The model under review builds one solid part; all positions refer to its coordinate system, in mm. Face numbers are marked on the shaded views. A direction names the side the tool comes from. Round coordinates to 2 decimals unless told otherwise and drop trailing zeros. Loops run counter-clockwise (first coordinate to the right, second up) from the corner with the lowest first, then second, coordinate; pieces in that order, holes last. Notation, with made-up numbers: M -34,56 L -8,56 A27 cw -8,81 Z; hole C -8,10 d9. An arc over 180 degrees is marked long. Answer as a JSON object with one key per item and string values. Group by question number.
Item 1: Consider section A-A (x = 0). Give the boundary of the cut face in (y, z) (3 decimals), and give its area (3 significant figures).
Item 2: Consider section B-B (z = 0). Give the boundary of the cut face in (x, y) (3 decimals), and give its area (3 significant figures).
Item 3: The part is to be moulded in two halves that separate along Z. For the marked faces 3, 4 and 5, say which applies: +Z half, -Z half, draft (parallel to the pull), parting line (faces both ways), or undercut.
Item 4: To check wall thickness, follow line 1 (Z direction, x = 0.25, y = 46.5); line 2 (X direction, y = -39.75, z = 0) (3 decimals); line 3 (X direction, y = 17, z = 0) (3 decimals). State the ranges of each line that lie inside material, in increasing order.
Item 5: Insertion check: P1, Ø1.5, axis at y = -24, z = -1, coming from the -X side; P2, Ø5, axis at x = 0, z = 0, coming from the -Y side; P3, Ø4, axis at y = -26, z = 4.5, coming from the -X side; P4, Ø2, axis at x = 2.5, z = 1, coming from the +Y side. Each pin has a flat end and moves straight along its axis. Give the tip position at first contact, or say it passes through.
Item 6: Consider section D-D (y = -2.5). Give the boundary of the cut face in (x, z) (3 decimals), and give its area (3 significant figures).
Item 7: Consider section C-C (y = 44.5). Give the boundary of the cut face in (x, z) (3 decimals).
Item 8: Tool access review of the marked faces 1 and 2: name each direction out of +Z, -Z, +X, -X, +Y, -Y from which nothing blocks a thin tool from reaching the whole face with its end or side.
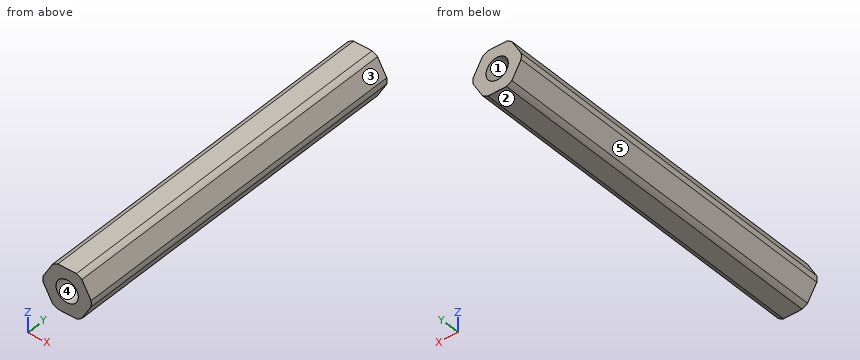
Autodesk Inventor part; units mm, degrees
ref_plane "YZ Plane" through (0, 0, 0) normal (1, 0, 0) x (0, 1, 0)
ref_plane "XZ Plane" through (0, 0, 0) normal (0, 1, 0) x (-1, 0, 0)
ref_plane "XY Plane" through (0, 0, 0) normal (0, 0, 1) x (1, 0, 0)
sketch "Sketch1" plane through (0, 0, 0) normal (0, 1, 0) x (-1, 0, 0)
  line L0 (-7.3323, 0) -> (-3.6662, 6.35)
  line L1 (-3.6662, 6.35) -> (3.6662, 6.35)
  line L2 (3.6662, 6.35) -> (7.3323, 0)
  line L3 (7.3323, 0) -> (3.6662, -6.35)
  line L4 (3.6662, -6.35) -> (-3.6662, -6.35)
  line L5 (-3.6662, -6.35) -> (-7.3323, 0)
  circle A0 centre (0, 0) radius 6.875
  circle A1 centre (0, 0) radius 6.35
  line L6 (-2.7496, -4.7625) -> (2.7496, -4.7625)
  line L7 (2.7496, -4.7625) -> (5.4993, 0)
  line L8 (5.4993, 0) -> (2.7496, 4.7625)
  line L9 (2.7496, 4.7625) -> (-2.7496, 4.7625)
  line L10 (-2.7496, 4.7625) -> (-5.4993, 0)
  line L11 (-5.4993, 0) -> (-2.7496, -4.7625)
  circle A2 centre (0, 0) radius 4.7625
  circle A3 centre (0, 0) radius 5.125
  circle A4 centre (0, 0) radius 9.525
  circle A5 centre (0, 0) radius 5.9436
  circle A6 centre (0, 0) radius 2.5527
  circle A7 centre (0, 0) radius 2.0193
  circle A8 centre (0, 0) radius 3.175
  circle A9 centre (0, 0) radius 8.7313
  point P0 (-4.1818, 5.457)
  point P1 (-2.635, 6.35)
  point P2 (-6.8168, -0.893)
  point P3 (-6.8168, 0.893)
  point P4 (-2.635, -6.35)
  point P5 (-4.1818, -5.457)
  point P6 (4.1818, -5.457)
  point P7 (2.635, -6.35)
  point P8 (6.8168, -0.893)
  point P9 (6.8168, 0.893)
  point P10 (2.635, 6.35)
  point P11 (4.1818, 5.457)
  point P12 (3.1778, -4.0208)
  point P13 (1.8932, -4.7625)
  point P14 (5.071, -0.7417)
  point P15 (5.071, 0.7417)
  point P16 (1.8932, 4.7625)
  point P17 (3.1778, 4.0208)
  point P18 (-3.1778, 4.0208)
  point P19 (-1.8932, 4.7625)
  point P20 (-5.071, -0.7417)
  point P21 (-5.071, 0.7417)
  point P22 (-1.8932, -4.7625)
  point P23 (-3.1778, -4.0208)
  dimension "d0" = 12.7
  dimension "d1" = 13.75
  dimension "d2" = 12.7
  dimension "d3" = 9.525
  dimension "d4" = 10.25
  dimension "d5" = 19.05
  dimension "d6" = 11.8872
  dimension "d7" = 5.1054
  dimension "d8" = 4.0386
  dimension "d9" = 6.35
  dimension "d153" = 0.7937
extrude "BaseProfile625Round" add sketch "Sketch1" along normal mid plane 101.6 contours L0 A0 L5 | A0 L0 | L0 A1 L5 A0 | L5 A0 | L0 A0 L1 A1 | A1 | L0 L1 A0 | A1 L4 A0 L5 | A0 L4 L5 | L1 A0 | L1 A0 L2 A1 | A1 L3 A0 L4 | L4 A0 | L1 L2 A0 | L2 A0 | L2 A0 L3 A1 | A0 L3 L4 | L3 A0 | L2 L3 A0 | L11 A3 L6 | A3 L11 A2 L6 | L6 A3 | A3 L11 | A2 L7 A3 L6 | A2 | A3 L7 L6 | L11 A3 L10 A2 | L11 L10 A3 | L7 A3 | A2 L8 A3 L7 | L10 A3 | L10 A3 L9 A2 | A3 L8 L7 | L10 L9 A3 | L9 A3 | L9 A3 L8 A2 | L8 A3 | L9 L8 A3 | A4 | A5 | A6 | A7 | A8 | A9
extrude "BaseProfileRoundTube" [suppressed]
extrude "BaseProfile500Hex" [suppressed]
extrude "BaseProfile500Thunderhex" cut sketch "Sketch1" along normal mid plane 914.4 contours L0 A0 L5 | A0 L0 | L5 A0 | L0 L1 A0 | A0 L4 L5 | L1 A0 | L4 A0 | L1 L2 A0 | L2 A0 | A0 L3 L4 | L3 A0 | L2 L3 A0 | A4 | A9
extrude "BaseProfile500Round" [suppressed]
extrude "BaseProfile375Hex" [suppressed]
extrude "BaseProfile375Thunderhex" [suppressed]
extrude "BaseProfile375Round" [suppressed]
extrude "TopShaftProfile1Hex500" [suppressed]
extrude "TopShaftProfile1ThunderHex500" [suppressed]
extrude "TopShaftProfile1Round500" [suppressed]
extrude "TopShaftProfile1Hex375" [suppressed]
extrude "TopShaftProfile1ThunderHex375" [suppressed]
extrude "TopShaftProfile1Round375" [suppressed]
extrude "TopShaftProfile2ThunderHex500" [suppressed]
extrude "TopShaftProfile2Round500" [suppressed]
extrude "TopShaftProfile2Hex375" [suppressed]
extrude "TopShaftProfile2ThunderHex375" [suppressed]
extrude "TopShaftProfile2Round375" [suppressed]
sketch "Sketch2" plane through (0, 0, 0) normal (1, 0, 0) x (0, 1, 0)
  line L0 (-92.7227, 0) -> (92.7227, 0)
  line L1 (0, -2.6658) -> (0, 15.9951)
  line L2 (50.8, 5.9436) -> (51.943, 5.9436)
  line L3 (51.943, 5.9436) -> (51.943, 6.35)
  line L4 (51.943, 6.35) -> (53.0225, 6.35)
  line L5 (53.0225, 6.35) -> (53.5305, 5.842)
  line L6 (53.5305, 5.842) -> (53.5305, 0)
  line L7 (50.8, 5.9436) -> (50.8, 0) construction
  line L8 (50.8, 5.9436) -> (50.8, 6.35)
  line L9 (50.8, 6.35) -> (50.8, 6.35)
  line L10 (50.8, 6.35) -> (50.8, 0)
  line L11 (50.8, 0) -> (53.5305, 0)
  line L12 (-50.8, 5.9436) -> (-51.943, 5.9436)
  line L13 (-51.943, 5.9436) -> (-51.943, 6.35)
  line L14 (-51.943, 6.35) -> (-53.0225, 6.35)
  line L15 (-53.0225, 6.35) -> (-53.5305, 5.842)
  line L16 (-53.5305, 5.842) -> (-53.5305, 0)
  line L17 (-50.8, 5.9436) -> (-50.8, 0) construction
  line L18 (-50.8, 5.9436) -> (-50.8, 6.35)
  line L19 (-50.8, 6.35) -> (-50.8, 6.35)
  line L20 (-50.8, 6.35) -> (-50.8, 0)
  line L21 (-50.8, 0) -> (-53.5305, 0)
  line L22 (0, 0) -> (0, 13.3292)
  line L23 (50.8, 0) -> (50.8, 6.35)
  point P0 (-53.5305, 0)
  point P1 (-50.8, 0)
  point P2 (30.955, 4.7625)
  point P3 (-17.4625, 6.2865)
  point P4 (25.4, 4.7625)
  point P5 (19.4005, 4.7625)
  point P6 (-25.4, 4.7625)
  point P7 (-26.543, 4.7625)
  dimension "TopBearingRoundDia2" = 12.7
  dimension "d65" = 45
  dimension "RetainingRingChamferSize2" = 0.508
  dimension "d72" = 50.8
  dimension "TopSnapRingDia2" = 11.8872
  dimension "d119" = 0.508
  dimension "d120" = 45
  dimension "d135" = 50.8
  dimension "d138" = 53.5305
  dimension "d139" = 51.943
  dimension "d140" = 50.8
  dimension "d141" = 11.8872
  dimension "d142" = 12.7
  dimension "d143" = 51.943
  dimension "d144" = 50.8
  dimension "d145" = 53.5305
revolve "TopRetentionGroove&BearingRound" [suppressed]
sketch "Sketch3" plane through (0, 50.8, 0) normal (0, 1, 0) x (1, 0, 0)
  point P0 (0, 0)
  point P1 (0, 0)
hole "TopShaftTappedHole" at (0, 50.8, 0) direction (0, -1, 0) diameter 6.35 depth 15.875 tip angle 118
thread "TopShaftThread"
extrude "BottomShaftProfile1Hex500" [suppressed]
extrude "BottomShaftProfile1ThunderHex500" [suppressed]
extrude "BottomShaftProfile1Round500" [suppressed]
extrude "BottomShaftProfile1Hex375" [suppressed]
extrude "BottomShaftProfile1ThunderHex375" [suppressed]
extrude "BottomShaftProfile2ThunderHex500" [suppressed]
extrude "BottomShaftProfile1Round375" [suppressed]
extrude "BottomShaftProfile2Round500" [suppressed]
extrude "BottomShaftProfile2Hex375" [suppressed]
extrude "BottomShaftProfile2ThunderHex375" [suppressed]
extrude "BottomShaftProfile2Round375" [suppressed]
sketch "Sketch4" plane through (0, -50.8, 0) normal (0, -1, 0) x (1, 0, 0)
  point P0 (0, 0)
  point P1 (0, 0)
hole "BottomShaftTappedHole" at (0, -50.8, 0) direction (0, 1, 0) diameter 6.35 depth 15.875 tip angle 118
thread "BottomShaftThread"
revolve "BottomRetentionGroove&BearingRound" [suppressed]
extrude "BaseProfile375ThunderhexHole" [suppressed]
extrude "BaseProfile500ThunderhexHole" cut sketch "Sketch1" along normal mid plane 914.4 contours A6 | A7
equation "\"d18\" = BottomShaftProfile1Depth + TopShaftProfile1Depth + BaseShaftLength + TopShaftProfile2Depth + BottomShaftProfile2Depth"
equation "\"d72\" = 0.5 * d18"
equation "\"BaseShaftLength\" = 101.6"
equation "\"TopShaftProfile1Depth\" = 0"
equation "\"TopShaftProfile2Depth\" = 0"
equation "\"BottomShaftProfile1Depth\" = 0"
equation "\"BottomShaftProfile2Depth\" = 0"
equation "\"TopShaftHoleDia\" = 6.35"
equation "\"BottomShaftHoleDia\" = 6.35"
equation "\"TopBearingRoundDia\" = 12.7"
equation "\"TopGrooveWidth\" = 1.143"
equation "\"TopBearingRoundDistance\" = 0"
equation "\"TopSnapRingDia\" = 11.8872"
equation "\"BottomBearingRoundDia\" = 12.7"
equation "\"BottomGrooveWidth\" = 1.143"
equation "\"BottomBearingRoundDistance\" = 0"
equation "\"BottomSnapRingDia\" = 11.8872"
equation "\"RoundTubeDia\" = 19.05"
equation "\"OrderLength\" = 114.3"
properties part number "217-4017, 4.5 in" material "Aluminum 7075"
Geometry results:
{
 "1": {"outline": "M -50.8,-6.35 L 50.8,-6.35 L 50.8,-3.175 L 34.925,-3.175 L 34.551,-2.553 L -34.551,-2.553 L -34.925,-3.175 L -50.8,-3.175 Z; M -50.8,3.175 L -34.925,3.175 L -34.551,2.553 L 34.551,2.553 L 34.925,3.175 L 50.8,3.175 L 50.8,6.35 L -50.8,6.35 Z", "area": "732 mm^2"},
 "2": {"outline": "M -6.875,-50.8 L -3.175,-50.8 L -3.175,-34.925 L -2.553,-34.551 L -2.553,34.551 L -3.175,34.925 L -3.175,50.8 L -6.875,50.8 Z; M 2.553,-34.551 L 3.175,-34.925 L 3.175,-50.8 L 6.875,-50.8 L 6.875,50.8 L 3.175,50.8 L 3.175,34.925 L 2.553,34.551 Z", "area": "838 mm^2"},
 "3": {"face 3": "+Z half", "face 4": "undercut", "face 5": "-Z half"},
 "4": {"line 1": "z = -6.35 to -3.17, 3.17 to 6.35", "line 2": "x = -6.875 to -3.175, 3.175 to 6.875", "line 3": "x = -6.875 to -2.553, 2.553 to 6.875"},
 "5": {"P1": "stops at x = -6.87", "P2": "passes through", "P3": "stops at x = -5.89", "P4": "stops at y = 50.8"},
 "6": {"outline": "M -6.817,-0.893 L -4.182,-5.457 A6.875 ccw -2.635,-6.35 L 2.635,-6.35 A6.875 ccw 4.182,-5.457 L 6.817,-0.893 A6.875 ccw 6.817,0.893 L 4.182,5.457 A6.875 ccw 2.635,6.35 L -2.635,6.35 A6.875 ccw -4.182,5.457 L -6.817,0.893 A6.875 ccw Z; hole C 0,0 d5.105", "area": "117 mm^2"},
 "7": {"outline": "M -6.817,-0.893 L -4.182,-5.457 A6.875 ccw -2.635,-6.35 L 2.635,-6.35 A6.875 ccw 4.182,-5.457 L 6.817,-0.893 A6.875 ccw 6.817,0.893 L 4.182,5.457 A6.875 ccw 2.635,6.35 L -2.635,6.35 A6.875 ccw -4.182,5.457 L -6.817,0.893 A6.875 ccw Z; hole C 0,0 d6.35"},
 "8": {"face 1": "+Y", "face 2": "-Z, +X, -X, +Y, -Y"}
}
